Autodesk Inventor part; units mm, degrees
ref_plane "Work Plane1" through (0, 3.25, 0) normal (0, -1, 0) x (1, 0, 0)
ref_plane "YZ Plane" through (0, 0, 0) normal (1, 0, 0) x (0, 1, 0)
ref_plane "XZ Plane" through (0, 0, 0) normal (0, 1, 0) x (-1, 0, 0)
sketch "Sketch1" plane through (0, 0, 0) normal (0, 0, 1) x (1, 0, 0)
  line L0 (0, 0) -> (20, 0)
  line L1 (20, 0) -> (20, 6.5)
  line L2 (20, 6.5) -> (0, 6.5)
  line L3 (0, 6.5) -> (0, 0)
  dimension "d0" = 20
  dimension "d1" = 6.5
extrude "Extrusion1" add sketch "Sketch1" along normal blind 10
sketch "Sketch2" plane through (0, 0, 10) normal (0, 0, 1) x (1, 0, 0)
  line L0 (3, 4.75) -> (4, 4.75)
  line L1 (4, 4.75) -> (4, 1.75)
  line L2 (4, 1.75) -> (3, 1.75)
  line L3 (3, 1.75) -> (3, 4.75)
  line L4 (0, 6.5) -> (0, 0)
  point P0 (3, 3.25)
  point P1 (0, 3.25)
  dimension "d4" = 1
  dimension "d5" = 3
  dimension "d6" = 3
extrude "Extrusion2" add sketch "Sketch2" along normal blind 1
sketch "Sketch3" plane through (0, 0, 0) normal (0, -1, 0) x (1, 0, 0)
  circle A0 centre (5, 3) radius 1.25
  circle A1 centre (15, 3) radius 1.25
  line L0 (5, 3) -> (15, 3) construction
  line L1 (0, 0) -> (20, 0) construction
  point P0 (10, 3)
  point P1 (10, 0)
  dimension "d9" = 2.5
  dimension "d10" = 2.5
  dimension "d11" = 3
  dimension "d12" = 10
extrude "Extrusion3" cut sketch "Sketch3" against normal through all
ref_plane "Work Plane1" through (0, 3.25, 0) normal (0, -1, 0) x (1, 0, 0)
sketch "Sketch4" plane through (0, 3.25, 0) normal (0, -1, 0) x (1, 0, 0)
  line L0 (0, 10) -> (-0.1016, 10.4)
  line L1 (-0.1016, 10.4) -> (24.1283, 16.5571)
  line L2 (24.1283, 16.5571) -> (24.2299, 16.1571)
  line L3 (24.2299, 16.1571) -> (0, 10)
  dimension "d15" = 0.4
  dimension "d19" = 25
extrude "Extrusion4" add sketch "Sketch4" along normal mid plane 4
properties part number "lever switch 20x10x6"
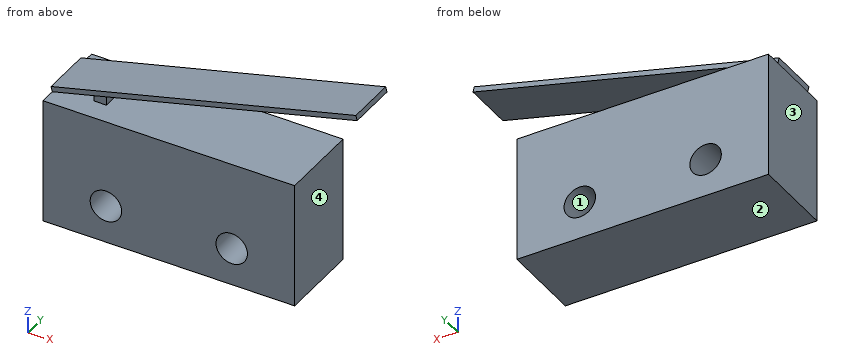
Geometry check sheet. Reference: the model listing, model coordinates, mm. Face numbers are marked on the shaded views. Coordinates: 2 decimals unless noted, no trailing zeros. Order: outer loops, then holes, each group sorted by start corner. A loop starts at its lowest first (then second) coordinate and runs counter-clockwise, first axis right, second up. Notation, with made-up numbers: (-10, 75) - (29, 75) arc R21 ccw to (29, 100) - close; hole circle Ø9 at (68, -24.5). An arc over 180 degrees is marked (long way). Answer as a JSON object with one key per item and string values. Group by question number.
Item 1: Depth check by flat-ended pin: pin 1 Ø1.1 at (y, z) = (2.5, 10.5) entering from +X; pin 2 Ø0.5 at (x, z) = (3.5, 10.5) entering from -Y; pin 3 Ø1 at (x, y) = (20.5, 4) entering from +Z. Enter the tip coordinate at first touch or a pass-through.
Item 2: Scan lines: probe 1 along Z at (x, y) = (5.75, 3.25); probe 2 along Z at (x, y) = (5, 3.75); probe 3 along X at (y, z) = (3.75, 6). Record each from-to range of solid material in increasing order.
Item 3: Sectioned sample at A-A, the plane z = 2.25. Record the cut outline in (x, y).
Item 4: Sectioned sample at B-B, the plane x = 8.25. Record the cut outline in (y, z), and give its area (3 significant figures).
Item 5: Sectioned sample at D-D, the plane x = 15.75. Record the cut outline in (y, z), and give its area (3 significant figures).
Item 6: Draft check along X on the marked faces 1, 2, 3 and 4. Enter one of: +X half, -X half, draft (parallel to the pull), parting line (faces both ways), or undercut.
Resolved:
{
 "1": {"pin 1": "x = 20", "pin 2": "y = 1.75", "pin 3": "z = 15.76"},
 "2": {"probe 1": "0 to 2, 4 to 10, 11.46 to 11.89", "probe 2": "0 to 1.75, 4.25 to 10, 11.27 to 11.7", "probe 3": "0 to 20"},
 "3": {"outline": "(0, 0) - (4, 0) - (4, 6.5) - (0, 6.5) - close; (6, 0) - (14, 0) - (14, 6.5) - (6, 6.5) - close; (16, 0) - (20, 0) - (20, 6.5) - (16, 6.5) - close"},
 "4": {"outline": "(0, 0) - (6.5, 0) - (6.5, 10) - (0, 10) - close; (1.25, 12.1) - (5.25, 12.1) - (5.25, 12.52) - (1.25, 12.52) - close", "area": "66.7 mm^2"},
 "5": {"outline": "(0, 0) - (6.5, 0) - (6.5, 2) - (0, 2) - close; (0, 4) - (6.5, 4) - (6.5, 10) - (0, 10) - close; (1.25, 14) - (5.25, 14) - (5.25, 14.43) - (1.25, 14.43) - close", "area": "53.7 mm^2"},
 "6": {"face 1": "undercut", "face 2": "draft", "face 3": "-X half", "face 4": "+X half"}
}
